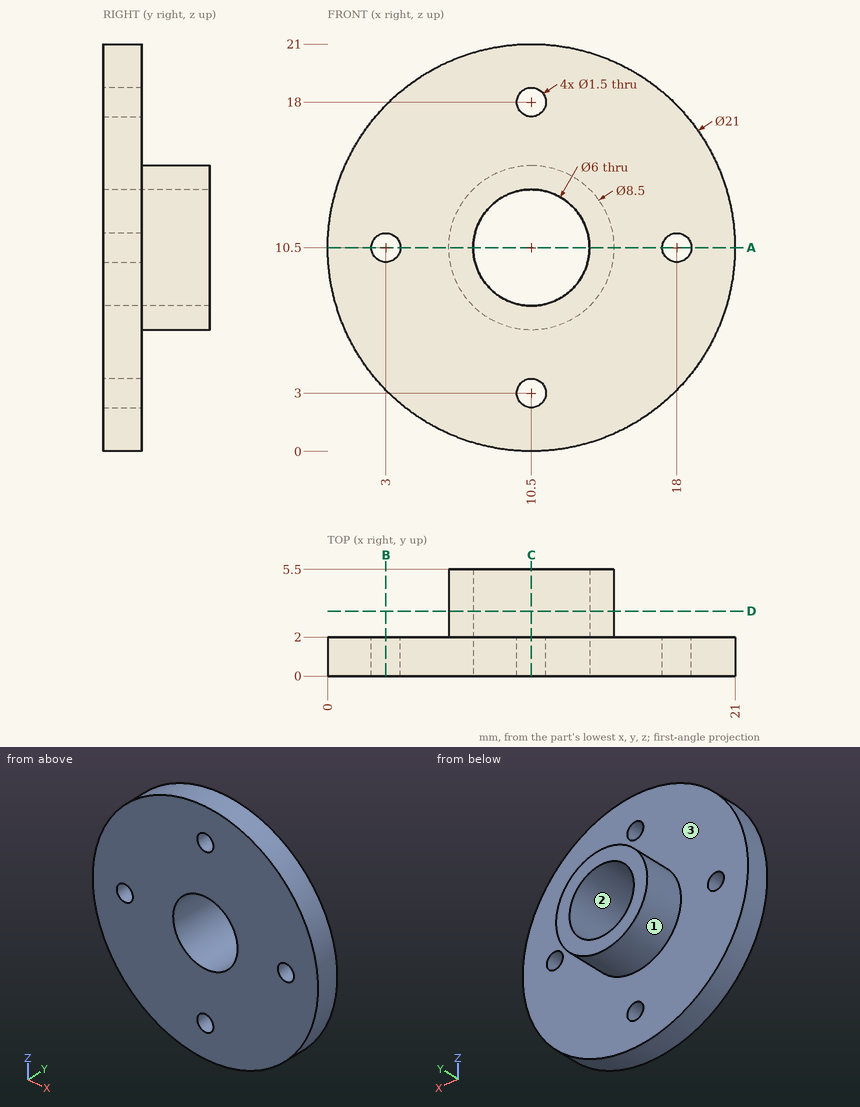
Print and shaded views of the part. All mm, measured from the part's lowest x, y and z. Coordinates: 2 decimals unless noted, no trailing zeros. Write each loop counter-clockwise with the first axis right and the second up, starting at its lowest first coordinate (ties: lowest second). Pieces come first, ordered by that corner, then holes. Notation, with made-up numbers: (-7, -20) - (48, -20) arc R17 cw to (48, -3) - close; hole circle Ø11 at (79.25, -3). An arc over 180 degrees is marked (long way). One line per question, with ' | ' between items. Start each with the question number.
Q1. Pull direction X, two halves, no side cores. Call the marked faces 1, 2 and 3: pulls with the +X half, pulls with the -X half, needs draft (parallel to the pull), parting line crosses it, or undercut.
Q2. Cut at B-B, the plane x = 3. List the corners of the cut face in (y, z), then the cut area to 3 significant figures.
Q3. Cut at A-A, the plane z = 10.5. List the corners of the cut face in (x, y), then the cut area to 4 significant figures.
Q4. Cut at C-C, the plane x = 10.5. List the corners of the cut face in (y, z).
Q5. Drill centre lines: line 1 (X direction, y = 1.55, z = 10.5); line 2 (Y direction, x = 4, z = 11.25); line 3 (X direction, y = 2.95, z = 8.25). Where is each one in solid material? Low to high. Write a range as [from, to].
Q6. Cut at D-D, the plane y = 3.35. List the corners of the cut face in (x, z).
Q7. Pin check, flat tips, straight feed: pin 1 (3.5 mm diameter, centred on x = 10.5, z = 10.5, fed in from +Y); pin 2 (3 mm diameter, centred on x = 14.5, y = 1.5, fed in from +Z); pin 3 (2 mm diameter, centred on y = 2.5, z = 8, fed in from -X); pin 4 (1 mm diameter, centred on x = 8.5, y = 3, fed in from -Z). Stop position of each tip, or through.
Answer below:
1) face 1: parting line crosses it | face 2: undercut | face 3: needs draft
2) outline: (0, 3.15) - (2, 3.15) - (2, 9.75) - (0, 9.75) - close; (0, 11.25) - (2, 11.25) - (2, 17.85) - (0, 17.85) - close | area: 26.4 mm^2
3) outline: (0, 0) - (2.25, 0) - (2.25, 2) - (0, 2) - close; (3.75, 0) - (7.5, 0) - (7.5, 5.5) - (6.25, 5.5) - (6.25, 2) - (3.75, 2) - close; (13.5, 0) - (17.25, 0) - (17.25, 2) - (14.75, 2) - (14.75, 5.5) - (13.5, 5.5) - close; (18.75, 0) - (21, 0) - (21, 2) - (18.75, 2) - close | area: 32.75 mm^2
4) outline: (0, 0) - (2, 0) - (2, 2.25) - (0, 2.25) - close; (0, 3.75) - (2, 3.75) - (2, 6.25) - (5.5, 6.25) - (5.5, 7.5) - (0, 7.5) - close; (0, 13.5) - (5.5, 13.5) - (5.5, 14.75) - (2, 14.75) - (2, 17.25) - (0, 17.25) - close; (0, 18.75) - (2, 18.75) - (2, 21) - (0, 21) - close
5) line 1: [0, 2.25], [3.75, 7.5], [13.5, 17.25], [18.75, 21] | line 2: [0, 2] | line 3: [6.89, 8.52], [12.48, 14.11]
6) outline: circle Ø8.5 at (10.5, 10.5); hole circle Ø6 at (10.5, 10.5)
7) pin 1: through | pin 2: z = 20.7 | pin 3: x = 0.13 | pin 4: z = 6.52
